Build history of the part. All positions in model axes, mm. Round coordinates to 2 decimals unless told otherwise and drop trailing zeros. Loops run counter-clockwise (first coordinate to the right, second up) from the corner with the lowest first, then second, coordinate; pieces in that order, holes last. Notation, with made-up numbers: M 5,12.25 L 50,12.25 A22 cw 50,28.25 Z; hole C 3.5,-32.5 d7. An arc over 180 degrees is marked long. One line per item, written item: value.
```python
from build123d import *

# Parameters (mm, degrees)
SKETCH1_R           = 25
SKETCH1_R_2         = 1.6
BOSS_EXTRUDE1_DEPTH = 1


with BuildPart() as part:
    # Sketch1 → Boss-Extrude1 (new body)
    with BuildSketch(Plane(origin=(0, 0, 0), x_dir=(0, 1, 0), z_dir=(0, 0, 1))):
        Circle(SKETCH1_R)
        with Locations((0, 11)):
            Circle(SKETCH1_R_2, mode=Mode.SUBTRACT)
        with Locations((11, 0)):
            Circle(SKETCH1_R_2, mode=Mode.SUBTRACT)
        with Locations((0, -11)):
            Circle(SKETCH1_R_2, mode=Mode.SUBTRACT)
        with Locations((-11, 0)):
            Circle(SKETCH1_R_2, mode=Mode.SUBTRACT)
    extrude(amount=BOSS_EXTRUDE1_DEPTH)


solid = part.part
```
Item 1: Slice it at D-D, the plane y = -11. Give the cut face in (x, z).
Check values:
outline: M -22.45,0 L -1.6,0 L -1.6,1 L -22.45,1 Z; M 1.6,0 L 22.45,0 L 22.45,1 L 1.6,1 Z
Item 2: Pull direction X, two halves, no side cores. Call faces 1 (the face through (-7.509, 23.846, 0.493)), 2 (the face through (0, 0, 0)), 3 (the face through (-0.07, -12.6, 0.49)): pulls with the +X half, pulls with the -X half, needs draft (parallel to the pull), parting line crosses it, or undercut.
Check values:
face 1: parting line crosses it
face 2: needs draft
face 3: undercut
Item 3: Slice it at A-A, the plane x = 0. Give the cut face in (y, z), and give its area (3 significant figures).
Check values:
outline: M -25,0 L -12.6,0 L -12.6,1 L -25,1 Z; M -9.4,0 L 9.4,0 L 9.4,1 L -9.4,1 Z; M 12.6,0 L 25,0 L 25,1 L 12.6,1 Z
area: 43.6 mm2
Item 4: Wall check: line 1 along Y through (x, z) = (0, 0.3); line 2 along X through (y, z) = (-1, 0.7). Give the ranges that are in metal, low to high.
Check values:
line 1: y = -25 to -12.6, -9.4 to 9.4, 12.6 to 25
line 2: x = -24.98 to -12.25, -9.75 to 9.75, 12.25 to 24.98
Item 5: Slice it at C-C, the plane z = 0.3. Give the cut face in (x, y), and give its area (3 significant figures).
Check values:
outline: C 0,0 d50; hole C -11,0 d3.2; hole C 0,-11 d3.2; hole C 0,11 d3.2; hole C 11,0 d3.2
area: 1,930 mm2
